Geometry: final body of the model. Coordinates: model frame, mm. A direction names the side the tool comes from. Give positions to 0.01 mm unless a question says otherwise; leave off trailing zeros. Order: outer loops, then holes, each group sorted by start corner. A loop starts at its lowest first (then second) coordinate and runs counter-clockwise, first axis right, second up. Notation, with made-up numbers: (-28.75, 31.5) -> (-15.75, 31.5) arc R10 cw to (-15.75, 37.5) -> close; hole circle Ø8 at (15.5, 60.5). An arc over 180 degrees is marked (long way). Write item = value, one per line.
```python
from build123d import *

# Parameters (mm, degrees)
SKETCH_1_W           = 55
SKETCH_1_H           = 39
EXTRUDE_1_DEPTH      = 2
SKETCH_2_W           = 23
SKETCH_2_H           = 6
EXTRUDE_2_DEPTH      = 2
SKETCH_3_W           = 6
SKETCH_3_H           = 5
EXTRUDE_3_DEPTH      = 11
SKETCH_5_R           = 0.95
CUT_EXTRUDE_1_DEPTH  = 11
SKETCH_6_W           = 55
SKETCH_6_H           = 0.171008225
EXTRUDE_4_DEPTH      = 8
SKETCH_8_R           = 1.65
EXTRUDE_6_DEPTH      = 2
SKETCH_10_W          = 3
SKETCH_10_H          = 6
EXTRUDE_7_DEPTH      = 8
SKETCH_11_R          = 1.5
CUT_EXTRUDE_3_DEPTH  = 13
SKETCH_12_R          = 3
EXTRUDE_8_DEPTH      = 7.5
SKETCH_13_W          = 10
SKETCH_13_H          = 3.7
EXTRUDE_9_DEPTH      = 1
FILLET_3_RADIUS      = 3
FILLET_3_LENGTH      = 3
SKETCH_15_R          = 1.75
CUT_EXTRUDE_5_DEPTH  = 23
SKETCH_16_W          = 15.5
SKETCH_16_H          = 4
EXTRUDE_10_DEPTH     = 20
SKETCH_17_R          = 1.5
EXTRUDE_11_DEPTH     = 10
FILLET_4_R           = 10
SKETCH_18_W          = 26.564734734
SKETCH_18_H          = 10.454508508
CUT_EXTRUDE_6_DEPTH  = 10
CUT_EXTRUDE_7_DEPTH  = 8
CUT_EXTRUDE_8_DEPTH  = 8
FILLET_6_R           = 5
SKETCH_22_R          = 1.4
CUT_EXTRUDE_10_DEPTH = 4


with BuildPart() as part:
    # 草图1 → 凸台-拉伸1 (new body)
    with BuildSketch(Plane(origin=(0, 0, 0), x_dir=(1, 0, 0), z_dir=(0, 1, 0))):
        Rectangle(SKETCH_1_W, SKETCH_1_H)
    extrude(amount=EXTRUDE_1_DEPTH)

    # 草图2 → 凸台-拉伸2 (add)
    with BuildSketch(Plane(origin=(0, 2, 0), x_dir=(1, 0, 0), z_dir=(0, 1, 0))):
        with Locations((0, -22.5)):
            Rectangle(SKETCH_2_W, SKETCH_2_H)
    extrude(amount=-EXTRUDE_2_DEPTH)

    # 草图3 → 凸台-拉伸3 (add)
    with BuildSketch(Plane(origin=(0, 2, 0), x_dir=(1, 0, 0), z_dir=(0, 1, 0))):
        with Locations((-9, -11.971008225)):
            Rectangle(SKETCH_3_W, SKETCH_3_H)
        with Locations((-9, 16.828991775)):
            Rectangle(SKETCH_3_W, SKETCH_3_H)
    extrude(amount=EXTRUDE_3_DEPTH)

    # 草图5 → 切除-拉伸1 (cut)
    with BuildSketch(Plane.ZY.offset(12)):
        with Locations((-16.278991775, 9.5)):
            Circle(SKETCH_5_R)
        with Locations((11.421008225, 9.5)):
            Circle(SKETCH_5_R)
    extrude(amount=-CUT_EXTRUDE_1_DEPTH, mode=Mode.SUBTRACT)

    # 草图6 → 凸台-拉伸4 (add)
    with BuildSketch(Plane(origin=(0, 2, 0), x_dir=(1, 0, 0), z_dir=(0, 1, 0))):
        with Locations((0, 19.414495888)):
            Rectangle(SKETCH_6_W, SKETCH_6_H)
    extrude(amount=EXTRUDE_4_DEPTH)

    # 草图8 → 凸台-拉伸6 (add, symmetric)
    with BuildSketch(Plane(origin=(0, 0, 0), x_dir=(0, 0, -1), z_dir=(1, 0, 0))):
        with BuildLine():
            Line((28.189872998, 17), (28.189872998, 0))
            Line((28.189872998, 0), (18.189872998, 0))
            Line((18.189872998, 0), (18.189872998, 17))
            ThreePointArc((18.189872998, 17), (23.189872998, 22), (28.189872998, 17))
        make_face()
        with Locations((23.189872998, 17)):
            Circle(SKETCH_8_R, mode=Mode.SUBTRACT)
    extrude(amount=EXTRUDE_6_DEPTH, both=True)

    # 草图10 → 凸台-拉伸7 (add)
    with BuildSketch(Plane(origin=(0, 2, 0), x_dir=(1, 0, 0), z_dir=(0, 1, 0))):
        with Locations((0, -20.5)):
            Rectangle(SKETCH_10_W, SKETCH_10_H)
    extrude(amount=EXTRUDE_7_DEPTH)

    # 草图11 → 切除-拉伸3 (cut)
    with BuildSketch(Plane.XY.offset(-19.328991775)):
        with Locations((-10, 3)):
            Circle(SKETCH_11_R)
    cut_extrude_3 = extrude(amount=-CUT_EXTRUDE_3_DEPTH, mode=Mode.SUBTRACT)

    # 草图12 → 凸台-拉伸8 (add)
    with BuildSketch(Plane.ZY.offset(27.5)):
        with BuildLine():
            Line((-39.5, -22), (-39.5, 10))
            Line((-39.5, 10), (-19.5, 10))
            Line((-19.5, 10), (-19.5, 0))
            Line((-19.5, 0), (-24.5, 0))
            Line((-24.5, 0), (-24.5, -22))
            ThreePointArc((-24.5, -22), (-32, -29.5), (-39.5, -22))
        make_face()
        with Locations((-32, -22)):
            Circle(SKETCH_12_R, mode=Mode.SUBTRACT)
    extrude_8 = extrude(amount=-EXTRUDE_8_DEPTH)

    # 草图13 → 凸台-拉伸9 (add)
    with BuildSketch(Plane.XZ):
        with Locations((0, 19.15)):
            Rectangle(SKETCH_13_W, SKETCH_13_H)
    extrude(amount=EXTRUDE_9_DEPTH)

    # 镜向1: 切除-拉伸3, 凸台-拉伸8 across plane
    add(cut_extrude_3.mirror(Plane(origin=(0, 0, 0), x_dir=(0, 0, 1), z_dir=(1, 0, 0))), mode=Mode.SUBTRACT)
    add(extrude_8.mirror(Plane(origin=(0, 0, 0), x_dir=(0, 0, 1), z_dir=(1, 0, 0))))

    # 圆角3: full round fillet: the end face becomes a half cylinder, R = half its width
    fillet_3_face = Plane((0, 10, 20.5), x_dir=(1, 0, 0), z_dir=(0, 1, 0))  # on the end face: x along it, z out of the body
    fillet_3_slab = fillet_3_face.offset(-FILLET_3_RADIUS / 2) * Box(FILLET_3_LENGTH, 2 * FILLET_3_RADIUS, FILLET_3_RADIUS, mode=Mode.PRIVATE)  # the body's end, R deep
    fillet_3_round = Plane((0, 7, 20.5), x_dir=(0, 1, 0), z_dir=(1, 0, 0)) * Cylinder(FILLET_3_RADIUS, FILLET_3_LENGTH, mode=Mode.PRIVATE)  # its axis R under the face
    add(fillet_3_slab - fillet_3_round, mode=Mode.SUBTRACT)

    # 草图15 → 切除-拉伸5 (cut)
    with BuildSketch(Plane.ZY.offset(1.5)):
        with Locations((20.5, 7)):
            Circle(SKETCH_15_R)
    extrude(amount=-CUT_EXTRUDE_5_DEPTH, mode=Mode.SUBTRACT)

    # 草图16 → 凸台-拉伸10 (add)
    with BuildSketch(Plane(origin=(0, 0, -19.5), x_dir=(-1, 0, 0), z_dir=(0, 0, -1))):
        with Locations((0, 8)):
            Rectangle(SKETCH_16_W, SKETCH_16_H)
    extrude(amount=EXTRUDE_10_DEPTH)

    # 草图17 → 凸台-拉伸11 (add)
    # profile 1 of 2: a face of its own
    with BuildSketch(Plane(origin=(0, 0, -19.5), x_dir=(-1, 0, 0), z_dir=(0, 0, -1))):
        Polygon((-20, 0), (-2, 0), (-2, 6), (-7.75, 6), (-7.75, 10), (-20, 10), align=None)
        with Locations(Location((-10, 3, 0), (0, 0, 221.810314896))):
            Circle(SKETCH_17_R, mode=Mode.SUBTRACT)
    # profile 2 of 2: a face of its own
    with BuildSketch(Plane(origin=(0, 0, -19.5), x_dir=(-1, 0, 0), z_dir=(0, 0, -1))):
        Polygon((7.75, 6), (2, 6), (2, 0), (20, 0), (20, 10), (7.75, 10), align=None)
        with Locations(Location((10, 3, 0), (0, 0, 180))):
            Circle(SKETCH_17_R, mode=Mode.SUBTRACT)
    extrude(amount=EXTRUDE_11_DEPTH)

    # 圆角4
    fillet_4_edges = [part.edges().sort_by_distance(p)[0] for p in [
        (23.75, 10, -39.5),
        (-23.75, 10, -39.5),
    ]]
    fillet(fillet_4_edges, radius=FILLET_4_R)

    # 草图18 → 切除-拉伸6 (cut)
    with BuildSketch(Plane(origin=(0, 10, 0), x_dir=(1, 0, 0), z_dir=(0, 1, 0))):
        with Locations((-0.840887807, 36.727254254)):
            Rectangle(SKETCH_18_W, SKETCH_18_H)
    extrude(amount=-CUT_EXTRUDE_6_DEPTH, mode=Mode.SUBTRACT)

    # 草图19 → 切除-拉伸7 (cut)
    with BuildSketch(Plane(origin=(27.5, 0, 0), x_dir=(0, 0, -1), z_dir=(1, 0, 0))):
        Polygon((24.3, 10), (39.5, -19.395601839), (39.5, 10), align=None)
    extrude(amount=-CUT_EXTRUDE_7_DEPTH, mode=Mode.SUBTRACT)

    # 草图20 → 切除-拉伸8 (cut)
    with BuildSketch(Plane.ZY.offset(27.5)):
        Polygon((-24.3, 10), (-39.5, 10), (-39.5, -19.395601839), align=None)
    extrude(amount=-CUT_EXTRUDE_8_DEPTH, mode=Mode.SUBTRACT)

    # 圆角6
    fillet_6_edges = [part.edges().sort_by_distance(p)[0] for p in [
        (-23.75, 0, -24.5),
        (23.75, 0, -24.5),
        (23.5, 10, -24.3),
        (-23.5, 10, -24.3),
    ]]
    fillet(fillet_6_edges, radius=FILLET_6_R)

    # 草图22 → 切除-拉伸10 (cut)
    with BuildSketch(Plane.XZ.offset(1)):
        with Locations(Location((0, 19.15, 0), (0, 0, 270))):
            Circle(SKETCH_22_R)
    extrude(amount=-CUT_EXTRUDE_10_DEPTH, mode=Mode.SUBTRACT)


solid = part.part
```
1) Section query B-B (y = -11). Output: boundary loops of the cut face in (x, z).
Check sheet entries:
outline = (-27.5, -35.16) -> (-20, -35.16) -> (-20, -24.5) -> (-27.5, -24.5) -> close; (20, -35.16) -> (27.5, -35.16) -> (27.5, -24.5) -> (20, -24.5) -> close
2) Section query C-C (x = 17.5). Output: boundary loops of the cut face in (y, z).
Check sheet entries:
outline = (0, -29.5) -> (10, -29.5) -> (10, -19.33) -> (2, -19.33) -> (2, 19.5) -> (0, 19.5) -> close
3) Section query D-D (z = 0.5). Output: boundary loops of the cut face in (x, y).
Check sheet entries:
outline = (-27.5, 0) -> (27.5, 0) -> (27.5, 2) -> (-27.5, 2) -> close
4) First-contact query: P1, Ø3.5, axis at x = 10, y = 3, coming from the -Z side; P2, Ø8, axis at x = -18, z = 10.5, coming from the +Y side; P3, Ø8, axis at x = -14.5, z = -6.5, coming from the -Y side; P4, Ø5.5, axis at y = -22, z = -32, coming from the +X side. Flat tips, straight axial feed; report the tip coordinate or a pass-through.
Check sheet entries:
P1 = -29.5
P2 = 2
P3 = 0
P4 = through
5) Section query A-A (x = -10). Output: boundary loops of the cut face in (y, z).
Check sheet entries:
outline = (0, -29.5) -> (1.5, -29.5) -> (1.5, -19.33) -> (4.5, -19.33) -> (4.5, -29.5) -> (10, -29.5) -> (10, -19.33) -> (13, -19.33) -> (13, -14.33) -> (2, -14.33) -> (2, 9.47) -> (13, 9.47) -> (13, 14.47) -> (2, 14.47) -> (2, 25.5) -> (0, 25.5) -> close; hole circle Ø1.9 at (9.5, -16.28); hole circle Ø1.9 at (9.5, 11.42)
6) Reachability of faces 1 (the face through (-11.5, 1, 23)), 2 (the face through (19, 1, 19.5)), 3 (the face through (-23.444, 9.291, -23.823)), 4 (the face through (-20, 6, -19.329)) from +Z, -Z, +X, -X, +Y, -Y: full face, straight path, thin tool, end or side. Return the list, or none.
Check sheet entries:
face_1 = +Z, -X, +Y, -Y
face_2 = +Z, +X, +Y, -Y
face_3 = -Z, -X, +Y
face_4 = +Z, -X, +Y
7) Line query: line 1 (X direction, y = 3, z = -26.75); line 2 (Y direction, x = -10, z = -21.75); line 3 (X direction, y = -11.5, z = -35). Output: solid intervals per line, ascending. Write a range as from..to.
Check sheet entries:
line_1 = -27.5..-11.5, -8.5..8.5, 11.5..27.5
line_2 = 0..1.5, 4.5..10
line_3 = -27.5..-20, 20..27.5
8) Mould query, pull axis Y, two halves, no side actions, for faces 5 (the face through (24, -22, -35)), 6 (the face through (0, 9, -18.19)), 7 (the face through (23.8, -29.5, -31.84)). Classes: +Y half, -Y half, draft (parallel to the pull), parting line (faces both ways), or undercut.
Check sheet entries:
face_5 = undercut
face_6 = draft
face_7 = -Y half
